The model under review builds one solid part; all positions refer to its coordinate system, in mm. Round coordinates to 2 decimals unless told otherwise and drop trailing zeros. Write each loop counter-clockwise with the first axis right and the second up, starting at its lowest first coordinate (ties: lowest second). Pieces come first, ordered by that corner, then holes.
Item 1: Add section B-B (x = -188.5). Give the boundary of the cut face in (y, z) (3 decimals), plus the area to 3 significant figures.
Item 2: Add section A-A (y = -3.75). Give the boundary of the cut face in (x, z).
Item 3: To check wall thickness, follow L1, parallel to Y at x = -38, z = -0.5; L2, parallel to Z at x = 135, y = 1; L3, parallel to Y at x = -160.5, z = -6.75. State the ranges of each line that lie inside material, in increasing order.
Item 4: Clearance check with flat-ended pins moving along their axes: pin 1 Ø3 at (y, z) = (6.5, 4) entering from -X; pin 2 Ø10 at (x, y) = (258.5, 8) entering from +Z; pin 3 Ø2 at (x, y) = (343.5, 8) entering from +Z; pin 4 Ø4 at (x, z) = (-81, 4) entering from +Y. State where each tip first meets the part, or that it passes through.
```python
from build123d import *

# Parameters (mm, degrees)
SKETCH1_R           = 11.525
SKETCH1_R_2         = 9.525
EXTRUDE_THIN1_DEPTH = 362.5
CUT_EXTRUDE1_DEPTH  = 23


with BuildPart() as part:
    # Sketch1 → Extrude-Thin1 (new, symmetric)
    with BuildSketch(Plane(origin=(0, 0, 0), x_dir=(0, 0, -1), z_dir=(1, 0, 0))):
        Circle(SKETCH1_R)
        Circle(SKETCH1_R_2, mode=Mode.SUBTRACT)
    extrude(amount=EXTRUDE_THIN1_DEPTH, both=True)

    # Sketch2 → Cut-Extrude1 (cut)
    with BuildSketch(Plane(origin=(0, 0, 0), x_dir=(1, 0, 0), z_dir=(0, 1, 0))):
        with BuildLine():
            Line((314.7, -6.35), (362.5, -6.35))
            Line((362.5, -6.35), (362.5, 6.35))
            Line((362.5, 6.35), (314.7, 6.35))
            ThreePointArc((314.7, 6.35), (312.578679656, 5.471320344), (311.7, 3.35))
            Line((311.7, 3.35), (311.7, -3.35))
            ThreePointArc((311.7, -3.35), (312.578679656, -5.471320344), (314.7, -6.35))
        make_face()
    cut_extrude1 = extrude(amount=CUT_EXTRUDE1_DEPTH, mode=Mode.SUBTRACT)

    # Mirror1: Cut-Extrude1 across plane
    add(cut_extrude1.mirror(Plane(origin=(0, 0, 0), x_dir=(0, 0, 1), z_dir=(1, 0, 0))), mode=Mode.SUBTRACT)


solid = part.part
```
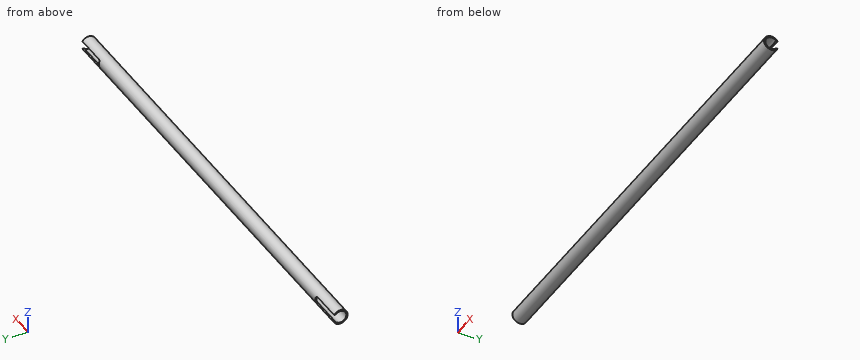
Numbers:
1. outline: circle Ø23.05 at (0, 0); hole circle Ø19.05 at (0, 0)
1. area: 132 mm2
2. outline: (-362.5, -10.9) - (362.5, -10.9) - (362.5, -8.76) - (-362.5, -8.76) - close; (-362.5, 8.76) - (362.5, 8.76) - (362.5, 10.9) - (-362.5, 10.9) - close
3. L1: y = -11.51 to -9.51, 9.51 to 11.51
3. L2: z = -11.48 to -9.47, 9.47 to 11.48
3. L3: y = -9.34 to -6.72, 6.72 to 9.34
4. pin 1: passes through
4. pin 2: stops at z = 11.13
4. pin 3: stops at z = 9.16
4. pin 4: stops at y = 11.35
